from build123d import *

# Parameters (mm, degrees)
SM_BASE_FLANGE_1_DEPTH = 100
SKETCH_6_W             = 23.5634
SKETCH_6_H             = 29
EXTRUDE_1_DEPTH        = 0.7
SKETCH_8_W             = 13.5634
SKETCH_8_H             = 80
EXTRUDE_3_DEPTH        = 0.7
SKETCH_9_R             = 3
CUT_EXTRUDE_1_DEPTH    = 0.7


# Sheet-metal steps are written as plain solids
with BuildPart() as part:
    # Sketch 1 → 基体-法兰1 (new body)
    with BuildSketch(Plane.XY):
        with BuildLine():
            Line((25, 29), (1.4366, 29))
            ThreePointArc((1.4366, 29), (0.420770398, 28.579229602), (0, 27.5634))
            Line((0, 27.5634), (0, 1.4366))
            ThreePointArc((0, 1.4366), (0.420770398, 0.420770398), (1.4366, 0))
            Line((1.4366, 0), (15, 0))
            Line((15, 0), (15, 0.7))
            Line((15, 0.7), (1.4366, 0.7))
            ThreePointArc((1.4366, 0.7), (0.915745145, 0.915745145), (0.7, 1.4366))
            Line((0.7, 1.4366), (0.7, 27.5634))
            ThreePointArc((0.7, 27.5634), (0.915745145, 28.084254855), (1.4366, 28.3))
            Line((1.4366, 28.3), (25, 28.3))
            Line((25, 28.3), (25, 29))
        make_face()
    extrude(amount=SM_BASE_FLANGE_1_DEPTH)

    # 草图6 → 凸台-拉伸1 (add)
    with BuildSketch(Plane(origin=(0, 29, 0), x_dir=(1, 0, 0), z_dir=(0, 1, 0))):
        with Locations((13.2183, 14.5)):
            Rectangle(SKETCH_6_W, SKETCH_6_H)
    extrude(amount=-EXTRUDE_1_DEPTH)

    # 草图8 → 凸台-拉伸3 (add)
    with BuildSketch(Plane.XZ):
        with Locations((8.2183, -40)):
            Rectangle(SKETCH_8_W, SKETCH_8_H)
    extrude(amount=-EXTRUDE_3_DEPTH)

    # 草图9 → 切除-拉伸1 (cut)
    with BuildSketch(Plane(origin=(0, 29, 0), x_dir=(1, 0, 0), z_dir=(0, 1, 0))):
        with Locations(Location((11.7, -90, 0), (0, 0, 270))):
            Circle(SKETCH_9_R)
        with Locations(Location((11.7, -10, 0), (0, 0, 270))):
            Circle(SKETCH_9_R)
    extrude(amount=-CUT_EXTRUDE_1_DEPTH, mode=Mode.SUBTRACT)


solid = part.part
The model under review builds one solid part; all positions refer to its coordinate system, in mm. A direction names the side the tool comes from. Round coordinates to 2 decimals unless told otherwise and drop trailing zeros. Write each loop counter-clockwise with the first axis right and the second up, starting at its lowest first coordinate (ties: lowest second). Pieces come first, ordered by that corner, then holes. Notation, with made-up numbers: M 16,-16 L 49,-16 A27 ccw 49,15 Z; hole C -39.75,36 d4. An arc over 180 degrees is marked long. Use a Markdown table: item, result. Add a question column.
Q1. The part is to be moulded in two halves that separate along X. For faces 4 (the face through (0.7, 14, 49)), 5 (the face through (13, 29, 35)), 6 (the face through (10.55, 28.65, 12.77)), say which applies: pulls with the +X half, pulls with the -X half, needs draft (parallel to the pull), parting line crosses it, or undercut.
Q2. We need section C-C, the plane x = 11.7. State the section outline as (y, z) points.
Q3. Machinability: for faces 1 (the face through (8, 0.7, 11)), 2 (the face through (0, 15, 49)), 3 (the face through (11.8, 28.7, 87)), which of the approach directions +Z, -Z, +X, -X, +Y, -Y give a long, thin tool a straight path to every point of the face, cutting with its end or side? Answer none if there is none.
Q4. Insertion check: pin 1 (1.1 mm diameter, centred on x = 1, y = 9.5, fed in from -Z); pin 2 (10 mm diameter, centred on x = 20.5, z = -9, fed in from -Y); pin 3 (0.8 mm diameter, centred on y = 0, z = -52, fed in from -X). Each pin has a flat end and moves straight along its axis. Give the tip position at first contact, or say it passes through.
Q5. To check wall thickness, follow line 1 (Y direction, x = 7.75, z = -17.5); line 2 (Y direction, x = 23, z = 83); line 3 (X direction, y = 28.7, z = 10). State the ranges of each line that lie inside material, in increasing order.
Q6. We need section D-D, the plane y = 18.5. State the section outline as (x, z) points.
Q7. We need section B-B, the plane z = 10. State the section outline as (x, y) points, plus the area to 3 significant figures.
Q8. We need section A-A, the plane x = 3.75. State the section outline as (y, z) points.
Findings below:
| question | item | result |
|---|---|---|
| 1 | face 4 | pulls with the +X half |
| 1 | face 5 | needs draft |
| 1 | face 6 | undercut |
| 2 | outline | M 0,-80 L 0.7,-80 L 0.7,100 L 0,100 Z; M 28.3,-29 L 29,-29 L 29,7 L 28.3,7 Z; M 28.3,13 L 29,13 L 29,87 L 28.3,87 Z; M 28.3,93 L 29,93 L 29,100 L 28.3,100 Z |
| 3 | face 1 | +Z, -Z, +X |
| 3 | face 2 | +Z, -Z, -X, +Y, -Y |
| 3 | face 3 | +Y |
| 4 | pin 1 | stops at z = 0 |
| 4 | pin 2 | stops at y = 28.3 |
| 4 | pin 3 | stops at x = 1.44 |
| 5 | line 1 | y = 0 to 0.7, 28.3 to 29 |
| 5 | line 2 | y = 28.3 to 29 |
| 5 | line 3 | x = 0.56 to 8.7, 14.7 to 25 |
| 6 | outline | M 0,0 L 0.7,0 L 0.7,100 L 0,100 Z |
| 7 | outline | M 0,1.44 A1.44 ccw 1.44,0 L 15,0 L 15,0.7 L 1.44,0.7 A0.74 cw 0.7,1.44 L 0.7,27.56 A0.74 cw 1.44,28.3 L 8.7,28.3 L 8.7,29 L 1.44,29 A1.44 ccw 0,27.56 Z; M 14.7,28.3 L 25,28.3 L 25,29 L 14.7,29 Z |
| 7 | area | 42.5 mm² |
| 8 | outline | M 0,-80 L 0.7,-80 L 0.7,100 L 0,100 Z; M 28.3,-29 L 29,-29 L 29,100 L 28.3,100 Z |
